Part model, mm, in its own coordinate system. Face numbers are marked on the shaded views. Give positions to 0.01 mm unless a question says otherwise; leave off trailing zeros. Return JSON: item names as keys, results as strings.
from build123d import *

# Parameters (mm, degrees)
F0_R     = 9.525
F0_R_2   = 5.08
F1_DEPTH = 12.7
F2_DEPTH = 25.4
F3_R     = 1.5875
F4_SIZE  = 1.5875


with BuildPart() as f1:
    # F0 (on Front) → F1 (new body)
    with BuildSketch(Plane.XZ):
        with BuildLine():
            ThreePointArc((4.1275, -18.597479), (14.858186, -11.922114), (19.05, 0))
            ThreePointArc((19.05, 0), (14.858186, 11.922114), (4.1275, 18.597479))
            ThreePointArc((4.1275, 18.597479), (-19.05, 0), (4.1275, -18.597479))
        make_face()
        Circle(F0_R, mode=Mode.SUBTRACT)
        with BuildLine():
            ThreePointArc((4.1275, 18.597479), (14.858186, 11.922114), (19.05, 0))
            ThreePointArc((19.05, 0), (14.858186, -11.922114), (4.1275, -18.597479))
            Line((4.1275, -18.597479), (40.438917, -10.538572))
            ThreePointArc((40.438917, -10.538572), (27.305, 0), (40.438917, 10.538572))
            Line((40.438917, 10.538572), (4.1275, 18.597479))
        make_face()
        with BuildLine():
            ThreePointArc((48.895, 0), (46.519639, 6.755865), (40.438917, 10.538572))
            ThreePointArc((40.438917, 10.538572), (27.305, 0), (40.438917, -10.538572))
            ThreePointArc((40.438917, -10.538572), (46.519639, -6.755865), (48.895, 0))
        make_face()
        with Locations((38.1, 0)):
            Circle(F0_R_2, mode=Mode.SUBTRACT)
    extrude(amount=F1_DEPTH)

    # F0 (on Front) → F2 (join)
    with BuildSketch(Plane.XZ):
        with BuildLine():
            ThreePointArc((4.1275, -18.597479), (14.858186, -11.922114), (19.05, 0))
            ThreePointArc((19.05, 0), (14.858186, 11.922114), (4.1275, 18.597479))
            ThreePointArc((4.1275, 18.597479), (-19.05, 0), (4.1275, -18.597479))
        make_face()
        Circle(F0_R, mode=Mode.SUBTRACT)
    extrude(amount=F2_DEPTH)

    # F3
    f3_edges = [f1.edges().sort_by_distance(p)[0] for p in [
        (-4.1275, -25.4, 18.597479),
        (-19.05, 0, 0),
        (22.283208, 0, 14.568026),
        (48.895, 0, 0),
        (22.283208, 0, -14.568026),
    ]]
    fillet(f3_edges, radius=F3_R)

    # F4
    f4_edges = [f1.edges().sort_by_distance(p)[0] for p in [
        (-9.525, -25.4, 0),
        (33.02, -12.7, 0),
    ]]
    chamfer(f4_edges, length=F4_SIZE)


solid = f1.part
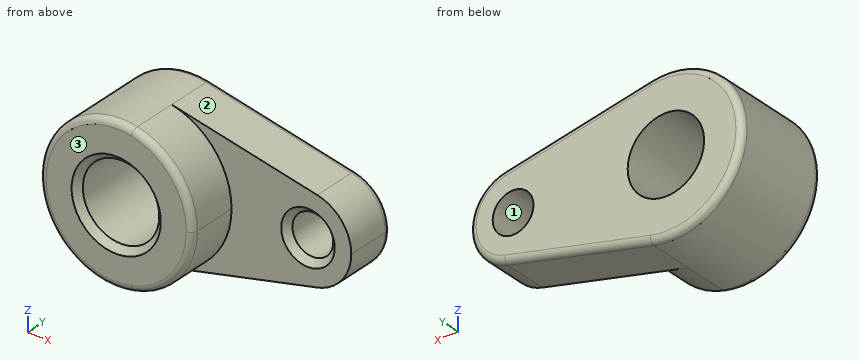
Q1. Probe line 1 along Z through (x, y) = (0, -17.75) (3 decimals); line 2 along X through (y, z) = (-4.75, -1); line 3 along Y through (x, z) = (42.5, -7). List the from-to ranges inside material, lowest first.
Established:
{"line 1": "z = -19.05 to -9.525, 9.525 to 19.05", "line 2": "x = -19.02 to -9.47, 9.47 to 33.12, 43.08 to 48.85", "line 3": "y = -12.7 to 0"}
Q2. Band-saw the part on A-A (y = -6.75). Give the number of separate pieces and of enclosed holes in the cut face, then the cut area to 3 significant figures.
Established:
{"separate pieces": "1", "enclosed holes": "2", "area": "1,550 mm²"}
Q3. Two-plate mould, pull along Z, no slides. Class the marked faces 1, 2 and 3: +Z half, -Z half, draft (parallel to the pull), parting line (faces both ways), or undercut.
Established:
{"face 1": "undercut", "face 2": "+Z half", "face 3": "draft"}
Q4. Pin check, flat tips, straight feed: pin 1 (10 mm diameter, centred on y = -3.5, z = -14, fed in from +X); pin 2 (13 mm diameter, centred on x = 38.1, z = 0, fed in from +Y); pin 3 (4 mm diameter, centred on x = 32.5, z = 13.5, fed in from +Y); pin 4 (1 mm diameter, centred on y = -8.5, z = -6, fed in from -X). Stop position of each tip, or through.
Established:
{"pin 1": "stops at x = 44.06", "pin 2": "stops at y = 0", "pin 3": "stops at y = -0.19", "pin 4": "stops at x = -18.24"}
